from build123d import *

# Parameters (mm, degrees)
F0_R           = 37.5
F1_DEPTH       = 3.86
F3_DEPTH       = 1
F5_D           = 4.4
F5_DEPTH       = 50
F5_CSINK_D     = 8.96
F5_CSINK_ANGLE = 90
F5_TIP         = 1.3218933619
F6_D           = 2.3
F6_DEPTH       = 50
F6_TIP         = 0.6909897119


# Not quite as in the source:
# - a feature names something its author has since deleted; it is built from what else it names


with BuildPart() as f1:
    # F0 (on Top) → F1 (new body)
    with BuildSketch(Plane.XY):
        Circle(F0_R)
        with BuildLine():
            Line((35.5279936079, -6.7726684482), (33.9669435175, -8.4407788788))
            ThreePointArc((33.9669435175, -8.4407788788), (24.9465264027, -24.5493547866), (8.9847812304, -33.8271149559))
            Line((8.9847812304, -33.8271149559), (7.0870357741, -35.7248604122))
            Line((7.0870357741, -35.7248604122), (5.8669428771, -34.5047675152))
            Line((5.8669428771, -34.5047675152), (2.7425574301, -31.3803820681))
            ThreePointArc((2.7425574301, -31.3803820681), (-22.2891525488, 22.2585641643), (31.3841187925, -2.6994606157))
            Line((31.3841187925, -2.6994606157), (34.5192493346, -5.7811266526))
            Line((34.5192493346, -5.7811266526), (35.5279936079, -6.7726684482))
        make_face(mode=Mode.SUBTRACT)
        with BuildLine():
            Line((28.6378246381, 0), (31.3841187925, -2.6994606157))
            ThreePointArc((31.3841187925, -2.6994606157), (-22.2891525488, 22.2585641643), (2.7425574301, -31.3803820681))
            Line((2.7425574301, -31.3803820681), (0, -28.6378246381))
            Line((0, -28.6378246381), (-28.6378246381, 0))
            Line((-28.6378246381, 0), (0, 28.6378246381))
            Line((0, 28.6378246381), (28.6378246381, 0))
        make_face()
        with BuildLine():
            Line((30.967620581, -5.7668427717), (26.7850823006, -1.8527423374))
            Line((26.7850823006, -1.8527423374), (1.8586698278, -26.7791548102))
            Line((1.8586698278, -26.7791548102), (6.2368967636, -30.8763844833))
            ThreePointArc((6.2368967636, -30.8763844833), (22.442510977, -22.1039295386), (30.967620581, -5.7668427717))
        make_face()
        with BuildLine():
            Line((33.9006451973, -8.5116240875), (30.967620581, -5.7668427717))
            ThreePointArc((30.967620581, -5.7668427717), (22.442510977, -22.1039295386), (6.2368967636, -30.8763844833))
            Line((6.2368967636, -30.8763844833), (9.1806708369, -33.6312253494))
            Line((9.1806708369, -33.6312253494), (8.9847812304, -33.8271149559))
            ThreePointArc((8.9847812304, -33.8271149559), (24.9465264027, -24.5493547866), (33.9669435175, -8.4407788788))
            Line((33.9669435175, -8.4407788788), (33.9006451973, -8.5116240875))
        make_face()
    extrude(amount=F1_DEPTH)

    # F2 (on face) → F3 (join)
    with BuildSketch(Plane.XY.offset(3.86)):
        with BuildLine():
            ThreePointArc((37.4966665185, -0.5), (37.4991666204, -0.250005556), (37.5, 0))
            ThreePointArc((37.5, 0), (37.4991666204, 0.250005556), (37.4966665185, 0.5))
            Line((37.4966665185, 0.5), (37.4966665185, -0.5))
        make_face()
        with BuildLine():
            Line((37.4966665185, -0.5), (37.4966665185, 0.5))
            ThreePointArc((37.4966665185, 0.5), (26.5165042945, 26.5165042945), (0.5, 37.4966665185))
            Line((0.5, 37.4966665185), (-0.5, 37.4966665185))
            ThreePointArc((-0.5, 37.4966665185), (-26.5165042945, 26.5165042945), (-37.4966665185, 0.5))
            Line((-37.4966665185, 0.5), (-37.4966665185, -0.5))
            ThreePointArc((-37.4966665185, -0.5), (-26.5165042945, -26.5165042945), (-0.5, -37.4966665185))
            Line((-0.5, -37.4966665185), (0.5, -37.4966665185))
            ThreePointArc((0.5, -37.4966665185), (26.5165042945, -26.5165042945), (37.4966665185, -0.5))
        make_face()
        with BuildLine():
            Line((-0.5, -27.0771644663), (-10.6461309606, -16.9310335056))
            ThreePointArc((-10.6461309606, -16.9310335056), (-5.7796293509, -19.1466938286), (-0.5, -19.9937490231))
            Line((-0.5, -19.9937490231), (-0.5, -27.0771644663))
        make_face(mode=Mode.SUBTRACT)
        with BuildLine():
            ThreePointArc((-19.9937490231, -0.5), (-19.1466938286, -5.7796293509), (-16.9310335056, -10.6461309606))
            Line((-16.9310335056, -10.6461309606), (-27.0771644663, -0.5))
            Line((-27.0771644663, -0.5), (-19.9937490231, -0.5))
        make_face(mode=Mode.SUBTRACT)
        with BuildLine():
            ThreePointArc((0.5, -19.9937490231), (5.7796293509, -19.1466938286), (10.6461309606, -16.9310335056))
            Line((10.6461309606, -16.9310335056), (0.5, -27.0771644663))
            Line((0.5, -27.0771644663), (0.5, -19.9937490231))
        make_face(mode=Mode.SUBTRACT)
        with BuildLine():
            Line((27.0771644663, -0.5), (16.9310335056, -10.6461309606))
            ThreePointArc((16.9310335056, -10.6461309606), (19.1466938286, -5.7796293509), (19.9937490231, -0.5))
            Line((19.9937490231, -0.5), (27.0771644663, -0.5))
        make_face(mode=Mode.SUBTRACT)
        with BuildLine():
            Line((-27.0771644663, 0.5), (-16.9310335056, 10.6461309606))
            ThreePointArc((-16.9310335056, 10.6461309606), (-19.1466938286, 5.7796293509), (-19.9937490231, 0.5))
            Line((-19.9937490231, 0.5), (-27.0771644663, 0.5))
        make_face(mode=Mode.SUBTRACT)
        with BuildLine():
            ThreePointArc((-0.5, 19.9937490231), (-5.7796293509, 19.1466938286), (-10.6461309606, 16.9310335056))
            Line((-10.6461309606, 16.9310335056), (-0.5, 27.0771644663))
            Line((-0.5, 27.0771644663), (-0.5, 19.9937490231))
        make_face(mode=Mode.SUBTRACT)
        with BuildLine():
            ThreePointArc((13.7885822494, 13.7885822168), (18.0156508884, 7.4623269205), (19.5, 0))
            ThreePointArc((19.5, 0), (18.015650884, -7.4623269311), (13.7885822331, -13.7885822331))
            ThreePointArc((13.7885822331, -13.7885822331), (4.88e-08, -19.5), (-13.7885821641, -13.7885823022))
            ThreePointArc((-13.7885821641, -13.7885823022), (-19.5, -3.62e-08), (-13.7885822154, 13.7885822509))
            ThreePointArc((-13.7885822154, 13.7885822509), (2.41e-08, 19.5), (13.7885822494, 13.7885822168))
        make_face(mode=Mode.SUBTRACT)
        with BuildLine():
            ThreePointArc((19.9937490231, 0.5), (19.1466938286, 5.7796293509), (16.9310335056, 10.6461309606))
            Line((16.9310335056, 10.6461309606), (27.0771644663, 0.5))
            Line((27.0771644663, 0.5), (19.9937490231, 0.5))
        make_face(mode=Mode.SUBTRACT)
        with BuildLine():
            Line((0.5, 27.0771644663), (10.6461309606, 16.9310335056))
            ThreePointArc((10.6461309606, 16.9310335056), (5.7796293509, 19.1466938286), (0.5, 19.9937490231))
            Line((0.5, 19.9937490231), (0.5, 27.0771644663))
        make_face(mode=Mode.SUBTRACT)
        with BuildLine():
            Line((-0.5, 37.4966665185), (0.5, 37.4966665185))
            ThreePointArc((0.5, 37.4966665185), (0, 37.5), (-0.5, 37.4966665185))
        make_face()
        with BuildLine():
            ThreePointArc((-0.5, -37.4966665185), (0, -37.5), (0.5, -37.4966665185))
            Line((0.5, -37.4966665185), (-0.5, -37.4966665185))
        make_face()
        with BuildLine():
            Line((-37.4966665185, -0.5), (-37.4966665185, 0.5))
            ThreePointArc((-37.4966665185, 0.5), (-37.5, 0), (-37.4966665185, -0.5))
        make_face()
    extrude(amount=F3_DEPTH)

    # F5
    with Locations(Plane.XY.offset(4.86)):
        with Locations((-20, -20), (20, -20), (20, 20), (-20, 20)):
            CounterSinkHole(F5_D / 2, F5_CSINK_D / 2, depth=F5_DEPTH, counter_sink_angle=F5_CSINK_ANGLE)
            with Locations((0, 0, -(F5_DEPTH + F5_TIP / 2))):  # 118° drill point
                Cone(0, F5_D / 2, F5_TIP, mode=Mode.SUBTRACT)

    # F6
    with Locations(Plane(origin=(0, 0, 0), x_dir=(1, 0, 0), z_dir=(0, 0, -1))):
        with Locations((-32.3357836379, -13.3939201328), (-13.3939201328, -32.3357836379), (13.3939201328, -32.3357836379), (32.3357836379, -13.3939201328), (32.3357836379, 13.3939201328), (13.3939201328, 32.3357836379), (-13.3939201328, 32.3357836379), (-32.3357836379, 13.3939201328)):
            Hole(F6_D / 2, depth=F6_DEPTH)
            with Locations((0, 0, -(F6_DEPTH + F6_TIP / 2))):  # 118° drill point
                Cone(0, F6_D / 2, F6_TIP, mode=Mode.SUBTRACT)


solid = f1.part
Source: CAD feature listing. Evaluate the final solid. Frame: model axes, mm. A direction names the side the tool comes from. Give positions to 0.01 mm unless a question says otherwise; leave off trailing zeros. Write each loop counter-clockwise with the first axis right and the second up, starting at its lowest first coordinate (ties: lowest second). Pieces come first, ordered by that corner, then holes. Notation, with made-up numbers: M 45,28 L 89,28 A30 ccw 89,66 Z; hole C 73,-30 d3. An arc over 180 degrees is marked long. Return JSON: item names as keys, results as strings. Group by question number.
1) Set-up query: faces 3 (the face through (-22.032, 19.157, 1.272)), 4 (the face through (14.12, 14.52, 1.9)). Return all of +Z, -Z, +X, -X, +Y, -Y with unobstructed straight access to the full face (end or side cutting, diameter ignored); none if empty.
2) Draft query along Y for faces 1 (the face through (-5.851, -19.125, 4.353)), 2 (the face through (16, -16, 4.86)). Return one class per face: released by +Y, released by -Y, zero draft, split by the parting line, or undercut.
3) Cut plane A-A, the plane z = 1.85. Give the number of separate pieces and of enclosed holes in the cut face, then the cut area to 3 significant figures.
4) Cut plane B-B, the plane x = -3. Output: boundary loops of the cut face in (y, z).
5) Ray query, L1, parallel to Y at x = 14, z = 1.9; L2, parallel to X at y = -6, z = 3; L3, parallel to Y at x = -23.5, z = 4.65. Return the intervals inside material, ascending.
6) First-contact query: pin 1 Ø0.8 at (y, z) = (23, 4.5) entering from -X; pin 2 Ø1.8 at (x, y) = (-13.39, -32.34) entering from -Z; pin 3 Ø6 at (x, y) = (-3.5, 29.5) entering from -Z; pin 4 Ø0.8 at (y, z) = (-24, 4.5) entering from +X. Flat tips, straight axial feed; report the tip coordinate or a pass-through.
Data:
{
 "1": {"face 3": "+Z, -Z", "face 4": "-Z"},
 "2": {"face 1": "undercut", "face 2": "zero draft"},
 "3": {"separate pieces": "1", "enclosed holes": "13", "area": "2,630 mm²"},
 "4": {"outline": "M -37.38,0 L -25.64,0 L -25.64,3.86 L -24.58,3.86 L -24.58,4.86 L -37.38,4.86 Z; M -19.77,3.86 L -19.27,3.86 L -19.27,4.86 L -19.77,4.86 Z; M 19.27,3.86 L 19.77,3.86 L 19.77,4.86 L 19.27,4.86 Z; M 24.58,3.86 L 25.64,3.86 L 25.64,0 L 37.38,0 L 37.38,4.86 L 24.58,4.86 Z"},
 "5": {"L1": "y = -34.79 to -33.31, -31.36 to -14.64, 14.64 to 31.36, 33.31 to 34.79", "L2": "x = -37.02 to -22.64, 22.64 to 31.22, 34.74 to 37.02", "L3": "y = -29.22 to -22.45, -17.55 to -4.08, -0.5 to 0.5, 4.08 to 17.55, 22.45 to 29.22"},
 "6": {"pin 1": "stops at x = -29.92", "pin 2": "passes through", "pin 3": "stops at z = 0", "pin 4": "stops at x = 29.14"}
}
